from build123d import *

# Parameters (mm, degrees)
F0_W      = 45
F0_H      = 77
F1_DEPTH  = 3
F4_DEPTH  = 11
F5_W      = 18
F5_H      = 15
F5_R      = 2.5
F6_DEPTH  = 14
F7_R      = 3
F8_R      = 5
F9_R      = 5
F11_DEPTH = 77.001


# Not quite as in the source:
# - a feature names something its author has since deleted; it is built from what else it names


with BuildPart() as f1:
    # F0 (on Top) → F1 (new body)
    with BuildSketch(Plane.XY):
        Rectangle(F0_W, F0_H)
    extrude(amount=F1_DEPTH)

    # F3 (on face) → F4 (join)
    with BuildSketch(Plane.XY.offset(3)):
        Polygon((19.5, -12.5), (22.5, -12.5), (22.5, 38.5), (-22.5, 38.5), (-22.5, 24.5), (-19.5, 24.5), (-19.5, 35.5), (19.5, 35.5), align=None)
        Polygon((22.5, -38.5), (22.5, -22.5), (19.5, -22.5), (19.5, -22.7520468089), (19.5, -35.5), (-19.5, -35.5), (-19.5, 9.5), (-22.5, 9.5), (-22.5, -38.5), align=None)
    extrude(amount=F4_DEPTH)

    # F5 (on Top) → F6 (join, through all)
    with BuildSketch(Plane.XY):
        with Locations((31.5, -1)):
            Rectangle(F5_W, F5_H)
        with Locations((33, -1)):
            Circle(F5_R, mode=Mode.SUBTRACT)
        with Locations((-31.5, -31)):
            Rectangle(F5_W, F5_H)
        with Locations((-33, -31)):
            Circle(F5_R, mode=Mode.SUBTRACT)
        with Locations((-31.5, -1)):
            Rectangle(F5_W, F5_H)
        with Locations((-33, -1)):
            Circle(F5_R, mode=Mode.SUBTRACT)
        with Locations((31.5, -31)):
            Rectangle(F5_W, F5_H)
        with Locations((33, -31)):
            Circle(F5_R, mode=Mode.SUBTRACT)
    extrude(amount=F6_DEPTH)

    # F7
    f7_edges = [f1.edges().sort_by_distance(p)[0] for p in [
        (-22.5, 38.5, 7),
        (22.5, 38.5, 7),
        (40.5, 6.5, 7),
        (40.5, -8.5, 7),
        (-40.5, 6.5, 7),
        (-40.5, -8.5, 7),
    ]]
    fillet(f7_edges, radius=F7_R)

    # F8
    f8_edges = [f1.edges().sort_by_distance(p)[0] for p in [
        (19.5, -35.5, 8.5),
        (-19.5, -35.5, 8.5),
        (19.5, 35.5, 8.5),
        (-19.5, 35.5, 8.5),
        (22.5, 6.5, 7),
        (22.5, -8.5, 7),
        (-22.5, -8.5, 7),
        (-22.5, 6.5, 7),
    ]]
    fillet(f8_edges, radius=F8_R)

    # F9
    f9_edges = [f1.edges().sort_by_distance(p)[0] for p in [
        (-40.5, -23.5, 7),
        (-22.5, -23.5, 7),
        (-40.5, -38.5, 7),
        (40.5, -38.5, 7),
        (40.5, -23.5, 7),
        (22.5, -23.5, 7),
    ]]
    fillet(f9_edges, radius=F9_R)

    # F10 (on face) → F11 (cut, through all)
    with BuildSketch(Plane.XZ.offset(38.5)):
        Polygon((-35.5, 0), (-25.5, 0), (-35.5, 3.6397023427), align=None)
        Polygon((-35.5, 0), (-35.5, 3.6397023427), (-49.4253699631, 8.7081225104), (-49.4253699631, 0), align=None)
        Polygon((35.5, 3.6397023427), (25.5, 0), (35.5, 0), align=None)
        Polygon((46.6463356366, 7.6966367355), (35.5, 3.6397023427), (35.5, 0), (46.6463356366, 0), align=None)
    extrude(amount=-F11_DEPTH, mode=Mode.SUBTRACT)


solid = f1.part
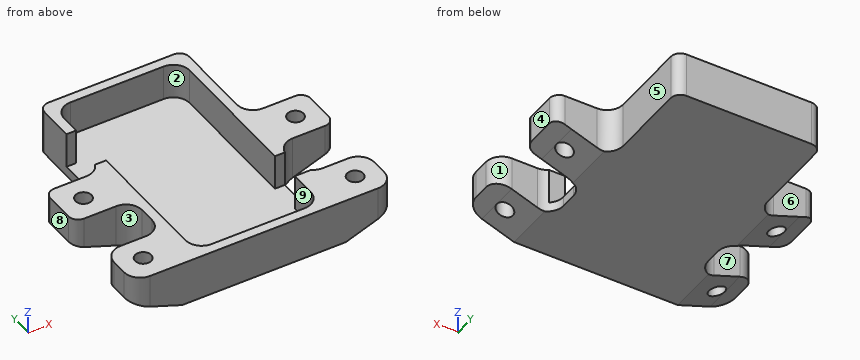
Geometry check sheet. Reference: the model listing, model coordinates, mm. Face numbers are marked on the shaded views. A direction names the side the tool comes from. Round coordinates to 2 decimals unless told otherwise and drop trailing zeros. Write each loop counter-clockwise with the first axis right and the second up, starting at its lowest first coordinate (ties: lowest second). Pieces come first, ordered by that corner, then holes. Notation, with made-up numbers: (78.25, 62) -> (88.25, 62) arc R25 cw to (88.25, 86) -> close; hole circle Ø1 at (31, 70.25). An arc over 180 degrees is marked (long way). One line per item, written item: value. Start each with the question number.
(1) Cross-section at C-C, the plane y = 28. Record the cut outline in (x, z).
(2) Cross-section at B-B, the plane x = 33. Record the cut outline in (y, z).
(3) Scan lines: line 1 (X direction, y = -1, z = 7.25); line 2 (Y direction, x = 33, z = 6.5); line 3 (X direction, y = 3, z = 6.75). Record each from-to range of solid material in increasing order. Write a range as [from, to].
(4) Cross-section at D-D, the plane x = -34. Record the cut outline in (y, z), and give its area (3 significant figures).
(5) Access from +Z, -Z, +X, -X, +Y, -Y to the whole of each face (thin tool, end or side, straight path). Record for the marked faces 1, 2, 3, 4 and 5.
(6) Draft check along Y on the marked faces 6, 7, 8 and 9. Enter one of: +Y half, -Y half, draft (parallel to the pull), parting line (faces both ways), or undercut.
(7) Go/stop test with flat-tipped pins: pin 1 Ø5 at (x, z) = (31.5, 6.5) entering from +Y; pin 2 Ø1.7 at (x, z) = (-21.5, 8.5) entering from +Y; pin 3 Ø1 at (y, z) = (14, 2.5) entering from +X; pin 4 Ø4.5 at (x, y) = (33, -1) entering from -Z. Record where each tip stops, or that it passes through.
(8) Cross-section at A-A, the plane y = -1. Record the cut outline in (x, z), and give its area (3 significant figures).
Answer:
1. outline: (-22.5, 0) -> (22.5, 0) -> (22.5, 14) -> (19.5, 14) -> (19.5, 3) -> (-19.5, 3) -> (-19.5, 14) -> (-22.5, 14) -> close
2. outline: (-38.5, 2.73) -> (-33.5, 2.73) -> (-33.5, 14) -> (-38.5, 14) -> close; (-28.5, 2.73) -> (-23.5, 2.73) -> (-23.5, 14) -> (-28.5, 14) -> close; (-8.5, 2.73) -> (-3.5, 2.73) -> (-3.5, 14) -> (-8.5, 14) -> close; (1.5, 2.73) -> (6.5, 2.73) -> (6.5, 14) -> (1.5, 14) -> close
3. line 1: [-40.5, -35.5], [-30.5, -19.5], [19.5, 30.5], [35.5, 40.5]
3. line 2: [-38.5, -33.5], [-28.5, -23.5], [-8.5, -3.5], [1.5, 6.5]
3. line 3: [-40.5, -19.5], [19.5, 40.5]
4. outline: (-38.5, 3.09) -> (-33.29, 3.09) -> (-33.29, 14) -> (-38.5, 14) -> close; (-28.71, 3.09) -> (-23.5, 3.09) -> (-23.5, 14) -> (-28.71, 14) -> close; (-8.5, 3.09) -> (-3.29, 3.09) -> (-3.29, 14) -> (-8.5, 14) -> close; (1.29, 3.09) -> (6.5, 3.09) -> (6.5, 14) -> (1.29, 14) -> close
4. area: 227 mm²
5. face 1: +Z, -Z, +X
5. face 2: +Z
5. face 3: +Z, -Z, -X
5. face 4: +Z, -Z, +X, +Y, -Y
5. face 5: +Z, -Z, +X, +Y
6. face 6: +Y half
6. face 7: undercut
6. face 8: draft
6. face 9: undercut
7. pin 1: y = 6.5
7. pin 2: y = 38.27
7. pin 3: x = 22.5
7. pin 4: through
8. outline: (-40.5, 5.46) -> (-35.5, 3.64) -> (-35.5, 14) -> (-40.5, 14) -> close; (-30.5, 1.82) -> (-25.5, 0) -> (25.5, 0) -> (30.5, 1.82) -> (30.5, 14) -> (19.5, 14) -> (19.5, 3) -> (-19.5, 3) -> (-19.5, 14) -> (-30.5, 14) -> close; (35.5, 3.64) -> (40.5, 5.46) -> (40.5, 14) -> (35.5, 14) -> close
8. area: 510 mm²
